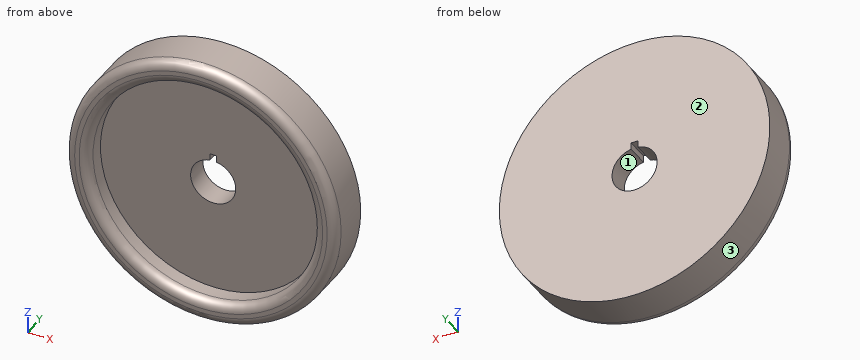
```python
from build123d import *

# Parameters (mm, degrees)
F0_R     = 76.2
F0_R_2   = 63.5
F1_DEPTH = 25.4
F2_DEPTH = 12.7
F3_R     = 5.08


with BuildPart() as f1:
    # F0 (on Front) → F1 (new body)
    with BuildSketch(Plane.XZ):
        Circle(F0_R)
        Circle(F0_R_2, mode=Mode.SUBTRACT)
    extrude(amount=F1_DEPTH)

    # F0 (on Front) → F2 (join)
    with BuildSketch(Plane.XZ):
        Circle(F0_R_2)
        with BuildLine():
            ThreePointArc((1.905, 12.556312), (0, -12.7), (-1.905, 12.556312))
            Line((-1.905, 12.556312), (-1.905, 16.366312))
            Line((-1.905, 16.366312), (1.905, 16.366312))
            Line((1.905, 16.366312), (1.905, 12.556312))
        make_face(mode=Mode.SUBTRACT)
    extrude(amount=F2_DEPTH)

    # F3
    f3_edges = [f1.edges().sort_by_distance(p)[0] for p in [
        (-76.2, -25.4, 0),
        (-63.5, -25.4, 0),
    ]]
    fillet(f3_edges, radius=F3_R)


solid = f1.part
```
Build history of the part. All positions in model axes, mm. Face numbers are marked on the shaded views. Give positions to 0.01 mm unless a question says otherwise; leave off trailing zeros. Loops run counter-clockwise (first coordinate to the right, second up) from the corner with the lowest first, then second, coordinate; pieces in that order, holes last.
1) Two-plate mould, pull along X, no slides. Class the marked faces 1, 2 and 3: released by +X, released by -X, zero draft, split by the parting line, or undercut.
Values follow:
face 1: undercut
face 2: zero draft
face 3: split by the parting line
2) Band-saw the part on A-A on z = 0. List the corners of the cut face in (x, y).
Values follow:
outline: (-76.2, -20.32) arc R5.08 ccw to (-71.12, -25.4) - (-68.58, -25.4) arc R5.08 ccw to (-63.5, -20.32) - (-63.5, -12.7) - (-12.7, -12.7) - (-12.7, 0) - (-76.2, 0) - close; (12.7, -12.7) - (63.5, -12.7) - (63.5, -20.32) arc R5.08 ccw to (68.58, -25.4) - (71.12, -25.4) arc R5.08 ccw to (76.2, -20.32) - (76.2, 0) - (12.7, 0) - close
3) Probe line 1 along Z through (x, y) = (0, -17.75); line 2 along Y through (x, z) = (26.5, 49); line 3 along X through (y, z) = (-12.75, -54.5). List the from-to ranges inside material, lowest first.
Values follow:
line 1: z = -76.2 to -63.5, 63.5 to 76.2
line 2: y = -12.7 to 0
line 3: x = -53.26 to -32.59, 32.59 to 53.26
4) Drop flat-ended pins along their axis: P1, Ø1, axis at x = -2.5, z = -45.5, coming from the -Y side; P2, Ø6, axis at y = -3.5, z = 10.5, coming from the +X side; P3, Ø8, axis at x = -47.5, y = -13, coming from the -Z side. Give the stop position or say it passes through.
Values follow:
P1: stops at y = -12.7
P2: stops at x = 75.83
P3: stops at z = -62.56
5) Band-saw the part on C-C on y = -5.5. List the corners of the cut face in (x, z) (3 decimals), then the cut area to 3 significant figures.
Values follow:
outline: circle Ø152.4 at (0, 0); hole (-1.905, 12.556) arc R12.7 ccw (long way) to (1.905, 12.556) - (1.905, 16.366) - (-1.905, 16.366) - close
area: 17,700 mm2
6) Band-saw the part on B-B on x = 0. List the corners of the cut face in (y, z), then the cut area to 3 significant figures.
Values follow:
outline: (-25.4, -71.12) arc R5.08 ccw to (-20.32, -76.2) - (0, -76.2) - (0, -12.7) - (-12.7, -12.7) - (-12.7, -63.5) - (-20.32, -63.5) arc R5.08 ccw to (-25.4, -68.58) - close; (-25.4, 68.58) arc R5.08 ccw to (-20.32, 63.5) - (-12.7, 63.5) - (-12.7, 16.37) - (0, 16.37) - (0, 76.2) - (-20.32, 76.2) arc R5.08 ccw to (-25.4, 71.12) - close
area: 1,870 mm2
